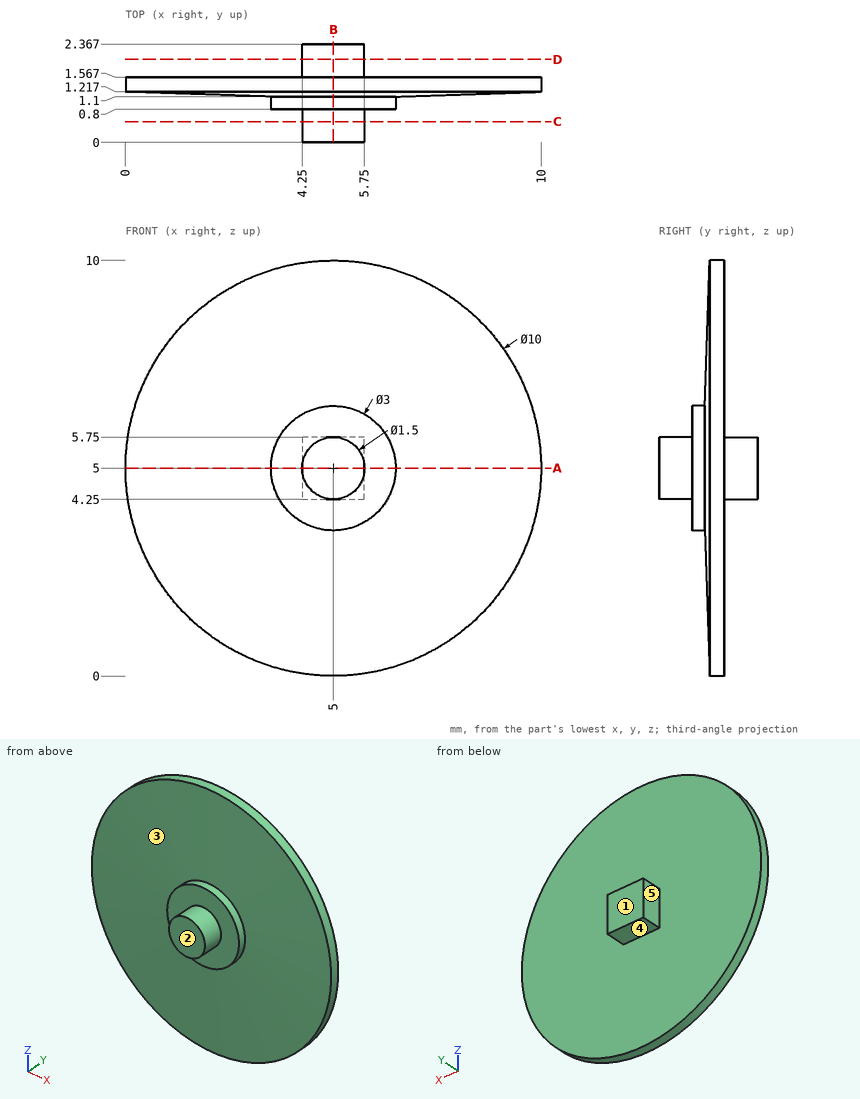
Here's the drawing with two shaded views (mm, measured from the low corner). I have some questions. A direction names the side the tool comes from. Coordinates: 2 decimals unless noted, no trailing zeros. Loops run counter-clockwise (first coordinate to the right, second up) from the corner with the lowest first, then second, coordinate; pieces in that order, holes last. Notation, with made-up numbers: M -22.5,-29.75 L -6.5,-29.75 A21 ccw -6.5,-1.75 Z; hole C 7.5,25.25 d3. An arc over 180 degrees is marked long. Put each result on its own line as item: value. Start each with the question number.
(1) Which directions (+Z, -Z, +X, -X, +Y, -Y) give clear straight access to the entire face, cutting with the end or side of a thin tool? Please do the marked faces 1, 2, 3, 4 and 5.
(2) I need wall thicknesses on probe 1 along X at (y, z) = (1.6, 4.5); probe 2 along Y at (x, z) = (5.75, 9); probe 3 along Z at (x, y) = (1.25, 1.3). Which ranges of each line are inside material? Lowest first, please.
(3) Will this pin go through, and if not, where does the flat tip stop? pin 1 Ø4 at (x, z) = (7.5, 8.5) entering from -Y.
(4) Imagine slicing it at A-A on z = 5. List the corners of the cut face in (x, y) for me.
(5) Imagine slicing it at D-D on y = 2. List the corners of the cut face in (x, z) for me, and give its area (3 significant figures).
(6) Imagine slicing it at C-C on y = 0.5. List the corners of the cut face in (x, z) for me.
(7) Imagine slicing it at B-B on x = 5. List the corners of the cut face in (y, z) for me.
Worked answers:
1. face 1: +Z, -Z, +X, -X, +Y
1. face 2: +Z, -Z, +X, -X, -Y
1. face 3: -Y
1. face 4: -Z, +X, -X, +Y
1. face 5: +Z, -Z, -X, +Y
2. probe 1: x = 4.25 to 5.75
2. probe 2: y = 1.19 to 1.57
2. probe 3: z = 1.69 to 8.31
3. pin 1: stops at y = 1.13
4. outline: M 0,1.22 L 3.5,1.1 L 3.5,0.8 L 4.25,0.8 L 4.25,0 L 5.75,0 L 5.75,0.8 L 6.5,0.8 L 6.5,1.1 L 10,1.22 L 10,1.57 L 5.75,1.57 L 5.75,2.37 L 4.25,2.37 L 4.25,1.57 L 0,1.57 Z
5. outline: M 4.25,4.25 L 5.75,4.25 L 5.75,5.75 L 4.25,5.75 Z
5. area: 2.25 mm2
6. outline: C 5,5 d1.5
7. outline: M 0,4.25 L 0.8,4.25 L 0.8,3.5 L 1.1,3.5 L 1.22,0 L 1.57,0 L 1.57,4.25 L 2.37,4.25 L 2.37,5.75 L 1.57,5.75 L 1.57,10 L 1.22,10 L 1.1,6.5 L 0.8,6.5 L 0.8,5.75 L 0,5.75 Z
